Read the model definition and answer for the solid it produces. Units are mm, in the model's axes. A direction names the side the tool comes from. Coordinates: 2 decimals unless noted, no trailing zeros. Write each loop counter-clockwise with the first axis right and the second up, starting at its lowest first coordinate (ties: lowest second). Pieces come first, ordered by that corner, then holes.
(1) The mould has two halves that part along X. Classify faces 4 (the flat face through (-35, 1, -17)), 5 (the flat face through (-17.3, 2, -5.6)), 6 (the flat face through (-17.65, 1.51, -6.24)), 7 (the flat face through (0, 1, -18)): +X half, -X half, draft (parallel to the pull), parting line (faces both ways), or undercut.
(2) Section C-C on z = -18 is taken. Write down the section's boundary in (x, y).
(3) Section A-A on x = -25.5 is taken. Write down the section's boundary in (y, z), then the cut area to 3 significant figures.
(4) Which of the six approach directions +Z, -Z, +X, -X, +Y, -Y give full straight-line access (tool end or side, diameter ignored) to faces 1 (the flat face through (-6, 0, -17)), 2 (the flat face through (-17.7, 0.5, -28.25)), 3 (the flat face through (-17.35, 1.51, -28.76))?
(5) Find the intervals of material crossed by probe 1 along X at (y, z) = (1.6, -12); probe 2 along Z at (x, y) = (-27, 1.5), in increasing order.
(6) Section B-B on y = 1.5 is taken. Write down the section's boundary in (x, z), then the cut area to 3 significant figures.
(7) Given pin 1 (6 mm diameter, centred on x = -7, z = -18.5, fed in from -Y), flat-ended and moving along its own axis, determine where the tip first touches the part or whether it passes through.
Autodesk Inventor part; units mm, degrees
ref_plane "YZ Plane" through (0, 0, 0) normal (1, 0, 0) x (0, 1, 0)
ref_plane "XZ Plane" through (0, 0, 0) normal (0, 1, 0) x (-1, 0, 0)
ref_plane "XY Plane" through (0, 0, 0) normal (0, 0, 1) x (1, 0, 0)
sketch "Sketch1" plane through (0, 0, 0) normal (0, 1, 0) x (-1, 0, 0)
  line L0 (0, 0) -> (35, 0)
  line L1 (35, 0) -> (35, -35)
  line L2 (35, -35) -> (0, -35)
  line L3 (0, -35) -> (0, 0)
  line L4 (6.75, -6.75) -> (28.25, -6.75)
  line L5 (28.25, -6.75) -> (28.25, -28.25)
  line L6 (28.25, -28.25) -> (6.75, -28.25)
  line L7 (6.75, -28.25) -> (6.75, -6.75)
  line L8 (6.75, -6.75) -> (28.25, -28.25) construction
  line L9 (28.25, -6.75) -> (6.75, -28.25) construction
  point P0 (17.5, -17.5)
  dimension "d0" = 35
  dimension "d1" = 35
  dimension "d2" = 21.5
  dimension "d3" = 21.5
extrude "Extrusion1" add sketch "Sketch1" along normal blind 2
chamfer "Chamfer1" distance 1 angle 45 2 edges at (-17.5, 2, -6.75) (-17.5, 2, -28.25)
properties part number "Plug_tester"
Response:
1. face 4: -X half
1. face 5: draft
1. face 6: undercut
1. face 7: +X half
2. outline: (-35, 0) - (-28.25, 0) - (-28.25, 2) - (-35, 2) - close; (-6.75, 0) - (0, 0) - (0, 2) - (-6.75, 2) - close
3. outline: (0, -35) - (2, -35) - (2, -29.25) - (1, -28.25) - (0, -28.25) - close; (0, -6.75) - (1, -6.75) - (2, -5.75) - (2, 0) - (0, 0) - close
3. area: 26.0 mm2
4. face 1: +Z, -Z, +X, -X, -Y
4. face 2: +Y, -Y
4. face 3: +Y
5. probe 1: x = -35 to -28.25, -6.75 to 0
5. probe 2: z = -35 to -28.75, -6.25 to 0
6. outline: (-35, -35) - (0, -35) - (0, 0) - (-35, 0) - close; hole (-28.25, -28.75) - (-6.75, -28.75) - (-6.75, -6.25) - (-28.25, -6.25) - close
6. area: 741 mm2
7. pin 1: stops at y = 0
